```python
from build123d import *

# Parameters (mm, degrees)
SKETCH1_R           = 1.45
BOSS_EXTRUDE1_DEPTH = 5.85
FILLET1_R           = 1
FILLET2_R           = 2.5


with BuildPart() as part:
    # Sketch1 → Boss-Extrude1 (new body)
    with BuildSketch(Plane(origin=(0, 0, 0), x_dir=(1, 0, 0), z_dir=(0, 1, 0))):
        with BuildLine():
            ThreePointArc((-26, 49), (-33.071067812, 46.071067812), (-36, 39))
            Line((-36, 39), (-36, 18.45))
            ThreePointArc((-36, 18.45), (-40.100505063, 8.550505063), (-50, 4.45))
            ThreePointArc((-50, 4.45), (-54.45, 0), (-50, -4.45))
            ThreePointArc((-50, -4.45), (-40.100505063, -8.550505063), (-36, -18.45))
            Line((-36, -18.45), (-36, -39))
            ThreePointArc((-36, -39), (-33.071067812, -46.071067812), (-26, -49))
            Line((-26, -49), (26, -49))
            ThreePointArc((26, -49), (33.071067812, -46.071067812), (36, -39))
            Line((36, -39), (36, -18.45))
            ThreePointArc((36, -18.45), (40.100505063, -8.550505063), (50, -4.45))
            ThreePointArc((50, -4.45), (54.45, 0), (50, 4.45))
            ThreePointArc((50, 4.45), (40.100505063, 8.550505063), (36, 18.45))
            Line((36, 18.45), (36, 39))
            ThreePointArc((36, 39), (33.071067812, 46.071067812), (26, 49))
            Line((26, 49), (-26, 49))
        make_face()
        Polygon((-23.5, -39), (0, -3.75), (23.5, -39), align=None, mode=Mode.SUBTRACT)
        Polygon((26, -35.25), (2.5, 0), (26, 35.25), align=None, mode=Mode.SUBTRACT)
        Polygon((23.5, 39), (0, 3.75), (-23.5, 39), align=None, mode=Mode.SUBTRACT)
        Polygon((-26, 35.25), (-2.5, 0), (-26, -35.25), align=None, mode=Mode.SUBTRACT)
        with Locations(Location((-50, 0, 0), (0, 0, 270))):
            Circle(SKETCH1_R, mode=Mode.SUBTRACT)
        with Locations(Location((0, 44, 0), (0, 0, 270))):
            Circle(SKETCH1_R, mode=Mode.SUBTRACT)
        with Locations(Location((50, 0, 0), (0, 0, 270))):
            Circle(SKETCH1_R, mode=Mode.SUBTRACT)
        with Locations(Location((0, -44, 0), (0, 0, 270))):
            Circle(SKETCH1_R, mode=Mode.SUBTRACT)
    extrude(amount=BOSS_EXTRUDE1_DEPTH)

    # Fillet1
    fillet1_edges = [part.edges().sort_by_distance(p)[0] for p in [
        (-23.5, 2.925, 39),
        (23.5, 2.925, 39),
        (23.5, 2.925, -39),
        (-23.5, 2.925, -39),
        (26, 2.925, 35.25),
        (26, 2.925, -35.25),
        (-26, 2.925, -35.25),
        (-26, 2.925, 35.25),
    ]]
    fillet(fillet1_edges, radius=FILLET1_R)

    # Fillet2
    fillet2_edges = [part.edges().sort_by_distance(p)[0] for p in [
        (0, 2.925, 3.75),
        (0, 2.925, -3.75),
        (2.5, 2.925, 0),
        (-2.5, 2.925, 0),
    ]]
    fillet(fillet2_edges, radius=FILLET2_R)


solid = part.part
```
The listing builds one solid part. Answer for the finished solid, in the listing's coordinates (mm). A direction names the side the tool comes from. Round coordinates to 2 decimals unless told otherwise and drop trailing zeros. Loops run counter-clockwise (first coordinate to the right, second up) from the corner with the lowest first, then second, coordinate; pieces in that order, holes last.
Q1. Section D-D, the plane z = 44 is taken. Determine the outline of the cut face in (x, y).
Q2. Which of the six approach directions +Z, -Z, +X, -X, +Y, -Y give full straight-line access (tool end or side, diameter ignored) to faces 1 (the face through (-26, 3, 0)), 2 (the face through (36, 3, -29)), 3 (the face through (36, 3, 29))?
Q3. Given pin 1 Ø2.5 at (x, z) = (0, 44) entering from -Y; pin 2 Ø3 at (y, z) = (3.5, 32) entering from +X; pin 3 Ø3 at (x, y) = (-33.5, 3.5) entering from -Z; pin 4 Ø3.5 at (x, z) = (0, -44) entering from -Y, each flat-ended and moving along its own axis, determine where each tip first touches the part or whether it passes through.
Q4. Section C-C, the plane x = 19.5 is taken. Determine the outline of the cut face in (y, z), then the cut area to 3 significant figures.
Q5. Section A-A, the plane z = 0 is taken. Determine the outline of the cut face in (x, y), then the cut area to 3 significant figures.
Q6. Section B-B, the plane x = 0 is taken. Determine the outline of the cut face in (y, z).
Q7. For a pull along X with two mould halves and no side action, classify faces 4 (the face through (0.06, 2.88, 42.55)), 5 (the face through (39.99, 2.88, 8.66)), 6 (the face through (-40.21, 2.88, 8.44)) as released by +X, released by -X, zero draft, split by the parting line, or undercut.
Q8. Find the intervals of material crossed by line 1 (X direction, y = 1.6, z = -22.5); line 2 (X direction, y = 1.3, z = 22); line 3 (Z direction, x = -18.5, y = 5.45), in increasing order.
Completed:
1. outline: (-34.66, 0) - (-1.45, 0) - (-1.45, 5.85) - (-34.66, 5.85) - close; (1.45, 0) - (34.66, 0) - (34.66, 5.85) - (1.45, 5.85) - close
2. face 1: +Y, -Y
2. face 2: -Z, +X, +Y, -Y
2. face 3: +Z, +X, +Y, -Y
3. pin 1: passes through
3. pin 2: stops at x = 36
3. pin 3: stops at z = -47
3. pin 4: stops at y = 0
4. outline: (0, -49) - (5.85, -49) - (5.85, -39) - (0, -39) - close; (0, -33) - (5.85, -33) - (5.85, -25.5) - (0, -25.5) - close; (0, 25.5) - (5.85, 25.5) - (5.85, 33) - (0, 33) - close; (0, 39) - (5.85, 39) - (5.85, 49) - (0, 49) - close
4. area: 205 mm2
5. outline: (-54.45, 0) - (-51.45, 0) - (-51.45, 5.85) - (-54.45, 5.85) - close; (-48.55, 0) - (-26, 0) - (-26, 5.85) - (-48.55, 5.85) - close; (-3, 0) - (3, 0) - (3, 5.85) - (-3, 5.85) - close; (26, 0) - (48.55, 0) - (48.55, 5.85) - (26, 5.85) - close; (51.45, 0) - (54.45, 0) - (54.45, 5.85) - (51.45, 5.85) - close
5. area: 334 mm2
6. outline: (0, -49) - (5.85, -49) - (5.85, -45.45) - (0, -45.45) - close; (0, -42.55) - (5.85, -42.55) - (5.85, -39) - (0, -39) - close; (0, -5.76) - (5.85, -5.76) - (5.85, 5.76) - (0, 5.76) - close; (0, 39) - (5.85, 39) - (5.85, 42.55) - (0, 42.55) - close; (0, 45.45) - (5.85, 45.45) - (5.85, 49) - (0, 49) - close
7. face 4: undercut
7. face 5: released by +X
7. face 6: released by -X
8. line 1: x = -36 to -26, -17.5 to -12.5, 12.5 to 17.5, 26 to 36
8. line 2: x = -36 to -26, -17.17 to -12.17, 12.17 to 17.17, 26 to 36
8. line 3: z = -49 to -39, -31.5 to -24, 24 to 31.5, 39 to 49
